```python
from build123d import *

# Parameters (mm, degrees)
SKETCH1_W                                         = 12.7
SKETCH1_H                                         = 50.8
BOSS_EXTRUDE1_DEPTH                               = 3.175
CSK_FOR_4_FLAT_HEAD_MACHINE_SCREW_100_D           = 3.2639
CSK_FOR_4_FLAT_HEAD_MACHINE_SCREW_100_CSINK_D     = 5.715
CSK_FOR_4_FLAT_HEAD_MACHINE_SCREW_100_CSINK_ANGLE = 100


with BuildPart() as part:
    # Sketch1 → Boss-Extrude1 (new, symmetric)
    with BuildSketch(Plane.XY):
        Rectangle(SKETCH1_W, SKETCH1_H)
    extrude(amount=BOSS_EXTRUDE1_DEPTH, both=True)

    # CSK for #4 Flat Head Machine Screw (100)1 (through all)
    with Locations(Plane.XY.offset(3.175)):
        with Locations((0, 12.7), (0, 0), (0, -12.7)):
            CounterSinkHole(CSK_FOR_4_FLAT_HEAD_MACHINE_SCREW_100_D / 2, CSK_FOR_4_FLAT_HEAD_MACHINE_SCREW_100_CSINK_D / 2, counter_sink_angle=CSK_FOR_4_FLAT_HEAD_MACHINE_SCREW_100_CSINK_ANGLE)


solid = part.part
```
Geometry: final body of the model. Coordinates: model frame, mm. Coordinates: 2 decimals unless noted, no trailing zeros. Write each loop counter-clockwise with the first axis right and the second up, starting at its lowest first coordinate (ties: lowest second). Pieces come first, ordered by that corner, then holes. Notation, with made-up numbers: M -38,18.25 L 20,18.25 A15 ccw 20,40.25 Z; hole C 70,2.25 d3. An arc over 180 degrees is marked long. Use CSV: the item, a comma, the result in double quotes. Start each with the question number.
1. Ray query, probe 1 along Y at (x, z) = (0, -1.9); probe 2 along Y at (x, z) = (0.75, -2.75); probe 3 along X at (y, z) = (12.7, -1.75). Return the intervals inside material, ascending.
2. Cut plane B-B on x = 0. Return the cut outline in (y, z) (1 decimal).
3. Mould query, pull axis Y, two halves, no side actions, for faces 1 (the face through (0.21, -11.08, -0.55)), 2 (the face through (3, 0, -3.175)), 3 (the face through (0, -25.4, 0)). Classes: pulls with the +Y half, pulls with the -Y half, needs draft (parallel to the pull), parting line crosses it, or undercut.
4. Cut plane C-C on z = -0.5. Return the cut outline in (x, y).
Entries:
1,probe 1,"-25.4 to -14.33, -11.07 to -1.63, 1.63 to 11.07, 14.33 to 25.4"
1,probe 2,"-25.4 to -14.15, -11.25 to -1.45, 1.45 to 11.25, 14.15 to 25.4"
1,probe 3,"-6.35 to -1.63, 1.63 to 6.35"
2,outline,"M -25.4,-3.2 L -14.3,-3.2 L -14.3,2.1 L -15.6,3.2 L -25.4,3.2 Z; M -11.1,-3.2 L -1.6,-3.2 L -1.6,2.1 L -2.9,3.2 L -9.8,3.2 L -11.1,2.1 Z; M 1.6,-3.2 L 11.1,-3.2 L 11.1,2.1 L 9.8,3.2 L 2.9,3.2 L 1.6,2.1 Z; M 14.3,-3.2 L 25.4,-3.2 L 25.4,3.2 L 15.6,3.2 L 14.3,2.1 Z"
3,face 1,"undercut"
3,face 2,"needs draft"
3,face 3,"pulls with the -Y half"
4,outline,"M -6.35,-25.4 L 6.35,-25.4 L 6.35,25.4 L -6.35,25.4 Z; hole C 0,-12.7 d3.26; hole C 0,0 d3.26; hole C 0,12.7 d3.26"
